from build123d import *

# Parameters (mm, degrees)
F0_R     = 4.3
F1_DEPTH = 5.15
F0_R_2   = 1.66
F2_DEPTH = 4
F3_DEPTH = 1.2


with BuildPart() as f1:
    # F0 (on Top) → F1 (new body)
    with BuildSketch(Plane.XY):
        with BuildLine():
            Line((5.5, -10.778409), (5.5, 0))
            ThreePointArc((5.5, 0), (3.080493, -4.556376), (-2.049295, -5.103958))
            ThreePointArc((-2.049295, -5.103958), (0.249491, -12.712308), (-5.5, -18.2))
            ThreePointArc((-5.5, -18.2), (-7.361798, -20.974231), (-4.839874, -23.165703))
            ThreePointArc((-4.839874, -23.165703), (-4.313128, -23.058356), (-3.791444, -22.928621))
            ThreePointArc((-3.791444, -22.928621), (2.910923, -18.426262), (5.5, -10.778409))
        make_face()
        with BuildLine():
            ThreePointArc((-2.049295, -5.103958), (3.080493, -4.556376), (5.5, 0))
            ThreePointArc((5.5, 0), (-3.080493, 4.556376), (-2.049295, -5.103958))
        make_face()
        Circle(F0_R, mode=Mode.SUBTRACT)
    extrude(amount=F1_DEPTH)

    # F0 (on Top) → F2 (join)
    with BuildSketch(Plane.XY):
        Circle(F0_R)
        Circle(F0_R_2, mode=Mode.SUBTRACT)
    extrude(amount=F2_DEPTH)

    # F0 (on Top) → F3 (cut)
    with BuildSketch(Plane.XY):
        Circle(F0_R)
        Circle(F0_R_2, mode=Mode.SUBTRACT)
    extrude(amount=F3_DEPTH, mode=Mode.SUBTRACT)


solid = f1.part
Model file for the job. Use its own axes, mm. A direction names the side the tool comes from. Give positions to 0.01 mm unless a question says otherwise; leave off trailing zeros. Order: outer loops, then holes, each group sorted by start corner. A loop starts at its lowest first (then second) coordinate and runs counter-clockwise, first axis right, second up. Notation, with made-up numbers: M 58,69.25 L 88,69.25 A34 cw 88,103.25 Z; hole C -18,64.25 d3. An arc over 180 degrees is marked long. Put each result on its own line as item: value. Start each with the question number.
(1) Drill centre lines: L1, parallel to Y at x = -1.5, z = 3.65; L2, parallel to Y at x = -3, z = 0.75; L3, parallel to Z at x = 1.25, y = 2.25. Where is each one in solid material? Low to high. Write a range as [from, to].
(2) Band-saw the part on C-C on x = 0. Give the cut face in (y, z).
(3) Band-saw the part on B-B on z = 0.7. Give the cut face in (x, y), then the cut area to 3 significant figures.
(4) Pin check, flat tips, straight feed: pin 1 Ø2.5 at (x, y) = (-0.5, 1.5) entering from +Z; pin 2 Ø3 at (x, z) = (-3.5, 1) entering from -Y; pin 3 Ø1 at (y, z) = (1, 1) entering from +X; pin 4 Ø1 at (y, z) = (-18.5, 4.5) entering from -X. Stop position of each tip, or through.
(5) Band-saw the part on A-A on x = -3. Give the cut face in (y, z).
(6) Tool access for faces 4 (the face through (0, -2, 4)), 5 (the face through (-4.32, -23.06, 2.54)), 6 (the face through (0, -2, 1.2)): list every direction of +Z, -Z, +X, -X, +Y, -Y with a clear straight run to the whole face (end or side of a thin tool).
(7) Band-saw the part on D-D on y = 3.75. Give the cut face in (x, z), then the cut area to 3 significant figures.
(8) Pull direction Y, two halves, no side cores. Call faces 1 (the face through (-7.37, -20.92, 2.54)), 2 (the face through (0.28, -12.6, 2.54)), 3 (the face through (2, -12, 5.15)): released by +Y, released by -Y, zero draft, split by the parting line, or undercut.
Results below:
1. L1: y = [-22.06, -15.91], [-5.64, -0.71], [0.71, 5.29]
1. L2: y = [-22.69, -17.17], [-4.61, -3.08], [3.08, 4.61]
1. L3: z = [1.2, 4]
2. outline: M -21.18,0 L -13.49,0 L -13.49,5.15 L -21.18,5.15 Z; M -8.07,0 L -4.3,0 L -4.3,1.2 L -1.66,1.2 L -1.66,4 L -4.3,4 L -4.3,5.15 L -8.07,5.15 Z; M 1.66,1.2 L 4.3,1.2 L 4.3,0 L 5.5,0 L 5.5,5.15 L 4.3,5.15 L 4.3,4 L 1.66,4 Z
3. outline: M -5.5,-18.2 A2.52 ccw -4.84,-23.17 A12.59 ccw -3.79,-22.93 A12.59 ccw 5.5,-10.78 L 5.5,0 A5.5 ccw long -2.05,-5.1 A7.59 cw Z; hole C 0,0 d8.6
3. area: 152 mm2
4. pin 1: stops at z = 4
4. pin 2: stops at y = -23.17
4. pin 3: stops at x = 5.48
4. pin 4: stops at x = -6.78
5. outline: M -22.69,0 L -17.17,0 L -17.17,5.15 L -22.69,5.15 Z; M -4.61,0 L -3.08,0 L -3.08,1.2 L 3.08,1.2 L 3.08,0 L 4.61,0 L 4.61,5.15 L 3.08,5.15 L 3.08,4 L -3.08,4 L -3.08,5.15 L -4.61,5.15 Z
6. face 4: +Z
6. face 5: +Z, -Z, +X, -Y
6. face 6: -Z
7. outline: M -4.02,0 L -2.1,0 L -2.1,1.2 L 2.1,1.2 L 2.1,0 L 4.02,0 L 4.02,5.15 L 2.1,5.15 L 2.1,4 L -2.1,4 L -2.1,5.15 L -4.02,5.15 Z
7. area: 31.6 mm2
8. face 1: split by the parting line
8. face 2: undercut
8. face 3: zero draft
